The model under review builds one solid part; all positions refer to its coordinate system, in mm. A direction names the side the tool comes from. Give positions to 0.01 mm unless a question says otherwise; leave off trailing zeros. Loops run counter-clockwise (first coordinate to the right, second up) from the corner with the lowest first, then second, coordinate; pieces in that order, holes last. Notation, with made-up numbers: M -26,73.25 L 30,73.25 A30 cw 30,99.25 Z; hole C -3,68.5 d2. An arc over 180 degrees is marked long. Put each result on its own line as item: value. Start each with the question number.
from build123d import *

# Parameters (mm, degrees)
SKETCH1_R           = 6
BOSS_EXTRUDE2_DEPTH = 12
BOSS_EXTRUDE3_DEPTH = 60
SKETCH3_R           = 6
CUT_EXTRUDE1_DEPTH  = 264.394047607


with BuildPart() as part:
    # Sketch1 → Boss-Extrude2 (new body)
    with BuildSketch(Plane(origin=(0, 0, 0), x_dir=(1, 0, 0), z_dir=(0, 1, 0))):
        with BuildLine():
            Line((400, 175), (400, 75))
            Line((400, 75), (290.473750966, 75))
            ThreePointArc((290.473750966, 75), (300, 0), (290.473750966, -75))
            Line((290.473750966, -75), (400, -75))
            Line((400, -75), (400, -175))
            Line((400, -175), (245.745613287, -172.072930905))
            Line((245.745613287, -172.072930905), (204.788011072, -143.394109088))
            ThreePointArc((204.788011072, -143.394109088), (250, 0), (204.788011072, 143.394109088))
            Line((204.788011072, 143.394109088), (245.745613287, 172.072930905))
            Line((245.745613287, 172.072930905), (400, 175))
        make_face()
        with Locations(Location((238.156986041, -137.5, 0), (0, 0, 270))):
            Circle(SKETCH1_R, mode=Mode.SUBTRACT)
        with Locations(Location((275, 0, 0), (0, 0, 270))):
            Circle(SKETCH1_R, mode=Mode.SUBTRACT)
        with Locations(Location((238.156986041, 137.5, 0), (0, 0, 270))):
            Circle(SKETCH1_R, mode=Mode.SUBTRACT)
    extrude(amount=BOSS_EXTRUDE2_DEPTH)

    # Sketch2 → Boss-Extrude3 (add)
    with BuildSketch(Plane(origin=(0, 12, 0), x_dir=(1, 0, 0), z_dir=(0, 1, 0))):
        Polygon((400, 75), (400, 175), (388.002159856, 174.772333819), (388.002159856, 75), align=None)
        Polygon((400, -175), (400, -75), (388.002159856, -75), (388.002159856, -174.772333819), align=None)
    extrude(amount=BOSS_EXTRUDE3_DEPTH)

    # Sketch3 → Cut-Extrude1 (cut, through all)
    with BuildSketch(Plane.ZY.offset(-388.002159856)):
        with Locations((-150, 42)):
            Circle(SKETCH3_R)
        with Locations((-100, 42)):
            Circle(SKETCH3_R)
        with Locations((100, 42)):
            Circle(SKETCH3_R)
        with Locations((150, 42)):
            Circle(SKETCH3_R)
    extrude(amount=-CUT_EXTRUDE1_DEPTH, mode=Mode.SUBTRACT)


solid = part.part
(1) To check wall thickness, follow L1, parallel to Y at x = 392.5, z = -100; L2, parallel to X at y = 30.5, z = -119; L3, parallel to Y at x = 293, z = -45. State the ranges of each line that lie inside material, in increasing order. Write a range as [from, to].
(2) We need section B-B, the plane y = 17. Write out the cut boundary in (x, z), plus the area to 3 significant figures.
(3) Draft analysis for pull direction X (two halves, no side actions). For faces 4 (the cylindrical face through (234.506, 5.916, 132.739)), 5 (the flat face through (394, 72, 124)), 6 (the flat face through (400, 35, 124)), state which applies: +X half, -X half, draft (parallel to the pull), parting line (faces both ways), or undercut.
(4) Insertion check: pin 1 (9.5 mm diameter, centred on x = 275, z = 0, fed in from -Y); pin 2 (6 mm diameter, centred on x = 246, z = -27.5, fed in from +Y); pin 3 (1.5 mm diameter, centred on y = 49.5, z = -101, fed in from -X); pin 4 (6 mm diameter, centred on y = 8.5, z = 44.5, fed in from +X). Each pin has a flat end and moves straight along its axis. Give the tip position at first contact, or say it passes through.
(5) We need section A-A, the plane z = 0. Write out the cut boundary in (x, y).
(6) We need section C-C, the plane z = 100. Write out the cut boundary in (x, y).
(7) For faces 1 (the flat face through (361.2, 11.8, -75)), 2 (the flat face through (298, 12, -2)), 3 (the flat face through (282, 0, -2)), list the 3-axis set-ups (+Z, -Z, +X, -X, +Y, -Y) from which the entire face can be reached by the end or side of a thin tool; tool diameter is ignored.
(8) We need section D-D, the plane z = -137.5. Write out the cut boundary in (x, y), plus the area to 3 significant figures.
Check sheet entries:
1. L1: y = [0, 36], [48, 72]
1. L2: x = [388, 400]
1. L3: y = [0, 12]
2. outline: M 388,-174.77 L 400,-175 L 400,-75 L 388,-75 Z; M 388,75 L 400,75 L 400,175 L 388,174.77 Z
2. area: 2,400 mm²
3. face 4: undercut
3. face 5: draft
3. face 6: +X half
4. pin 1: passes through
4. pin 2: stops at y = 12
4. pin 3: stops at x = 388
4. pin 4: stops at x = 297.12
5. outline: M 250,0 L 269,0 L 269,12 L 250,12 Z; M 281,0 L 300,0 L 300,12 L 281,12 Z
6. outline: M 229.13,0 L 400,0 L 400,36 L 388,36 L 388,12 L 229.13,12 Z; M 388,48 L 400,48 L 400,72 L 388,72 Z
7. face 1: +X, +Y, -Y
7. face 2: +Z, -Z, -X, +Y
7. face 3: +Z, -Z, +X, -X, -Y
8. outline: M 208.79,0 L 232.16,0 L 232.16,12 L 208.79,12 Z; M 244.16,0 L 400,0 L 400,72 L 388,72 L 388,12 L 244.16,12 Z
8. area: 2,870 mm²
